```python
from build123d import *

# Parameters (mm, degrees)
SKETCH1_W           = 12
SKETCH1_H           = 12
BOSS_EXTRUDE1_DEPTH = 3
SHELL2_T            = -1.8
SKETCH3_R           = 1.5
CUT_EXTRUDE3_DEPTH  = 1.8
BOSS_EXTRUDE2_START = 2
SKETCH3_3_W         = 16
SKETCH3_3_H         = 16
SKETCH3_3_W_2       = 12
SKETCH3_3_H_2       = 12
SKETCH3_3_R         = 1.5
BOSS_EXTRUDE2_DEPTH = 2
SKETCH4_W           = 14
SKETCH4_H           = 2
BOSS_EXTRUDE3_DEPTH = 2
SKETCH5_W           = 16
SKETCH5_H           = 16
SKETCH5_W_2         = 12
SKETCH5_H_2         = 12
BOSS_EXTRUDE4_DEPTH = 3
SKETCH6_W           = 14
SKETCH6_H           = 5
CUT_EXTRUDE4_DEPTH  = 2
SKETCH7_W           = 12
SKETCH7_H           = 5
CUT_EXTRUDE5_DEPTH  = 2
CUT_EXTRUDE6_DEPTH  = 0.5
SKETCH9_R           = 0.8
CUT_EXTRUDE7_DEPTH  = 21.420577881


with BuildPart() as part:
    # Sketch1 → Boss-Extrude1 (new body)
    with BuildSketch(Plane(origin=(0, 0, 0), x_dir=(1, 0, 0), z_dir=(0, 1, 0))):
        with Locations((6, -6)):
            Rectangle(SKETCH1_W, SKETCH1_H)
    extrude(amount=-BOSS_EXTRUDE1_DEPTH)

    # Shell2
    shell2_openings = [part.faces().sort_by_distance(p)[0] for p in [
        (6, -3, 6),
    ]]
    offset(amount=SHELL2_T, openings=shell2_openings, kind=Kind.INTERSECTION)

    # Sketch3 → Cut-Extrude3 (cut)
    with BuildSketch(Plane(origin=(0, 0, 0), x_dir=(1, 0, 0), z_dir=(0, 1, 0))):
        with Locations(Location((6, -6, 0), (0, 0, 270))):
            Circle(SKETCH3_R)
    extrude(amount=-CUT_EXTRUDE3_DEPTH, mode=Mode.SUBTRACT)

    # Sketch3<3> → Boss-Extrude2 (add)
    # profile 1 of 2: a face of its own
    with BuildSketch(Plane(origin=(0, 0, 0), x_dir=(1, 0, 0), z_dir=(0, 1, 0)).offset(BOSS_EXTRUDE2_START)):
        with Locations((6, -6)):
            Rectangle(SKETCH3_3_W, SKETCH3_3_H)
        with Locations((6, -6)):
            Rectangle(SKETCH3_3_W_2, SKETCH3_3_H_2, mode=Mode.SUBTRACT)
    # profile 2 of 2: a face of its own
    with BuildSketch(Plane(origin=(0, 0, 0), x_dir=(1, 0, 0), z_dir=(0, 1, 0)).offset(BOSS_EXTRUDE2_START)):
        with Locations((6, -6)):
            Rectangle(SKETCH3_3_W_2, SKETCH3_3_H_2)
        with Locations(Location((6, -6, 0), (0, 0, 270))):
            Circle(SKETCH3_3_R, mode=Mode.SUBTRACT)
    extrude(amount=-BOSS_EXTRUDE2_DEPTH)

    # Sketch4 → Boss-Extrude3 (add)
    with BuildSketch(Plane(origin=(0, 2, 0), x_dir=(1, 0, 0), z_dir=(0, 1, 0))):
        Polygon((0, 2), (-2, 2), (-2, -14), (0, -14), (0, 0), align=None)
        with Locations((7, 1)):
            Rectangle(SKETCH4_W, SKETCH4_H)
    extrude(amount=BOSS_EXTRUDE3_DEPTH)

    # Sketch5 → Boss-Extrude4 (add)
    with BuildSketch(Plane.XZ):
        with Locations((6, 6)):
            Rectangle(SKETCH5_W, SKETCH5_H)
        with Locations((6, 6)):
            Rectangle(SKETCH5_W_2, SKETCH5_H_2, mode=Mode.SUBTRACT)
    extrude(amount=BOSS_EXTRUDE4_DEPTH)

    # Sketch6 → Cut-Extrude4 (cut)
    with BuildSketch(Plane.XY.offset(14)):
        with Locations((7, -0.5)):
            Rectangle(SKETCH6_W, SKETCH6_H)
    extrude(amount=-CUT_EXTRUDE4_DEPTH, mode=Mode.SUBTRACT)

    # Sketch7 → Cut-Extrude5 (cut)
    with BuildSketch(Plane(origin=(14, 0, 0), x_dir=(0, 0, -1), z_dir=(1, 0, 0))):
        with Locations((-6, -0.5)):
            Rectangle(SKETCH7_W, SKETCH7_H)
    extrude(amount=-CUT_EXTRUDE5_DEPTH, mode=Mode.SUBTRACT)

    # Sketch8 → Cut-Extrude6 (cut)
    with BuildSketch(Plane.XY.offset(12)):
        with BuildLine():
            Line((5.499365182, -0.030316533), (6.944147055, 0.139116978))
            add(Edge.make_bspline(
                [(6.944147055, 0.139116978), (7.033959338, 0.149589911), (7.207292534, 0.169802147), (7.456935343, 0.206659273), (7.686554115, 0.246864239), (7.896440991, 0.291462829), (8.086108286, 0.339865769), (8.256388111, 0.390049541), (8.406137381, 0.446305372), (8.496905896, 0.49005931), (8.539974305, 0.51081995)],
                knots=[0, 0, 0, 0, 1.318163599, 2.543989528, 3.678365744, 4.716171039, 5.671329954, 6.531514493, 7.303223867, 8, 8, 8, 8], degree=3))
            Line((8.539974305, 0.51081995), (8.894602583, 0.146997606))
            add(Edge.make_bspline(
                [(8.894602583, 0.146997606), (8.903504519, 0.13774703), (8.91939642, 0.121232731), (8.933040884, 0.094560662), (8.942770969, 0.072093955), (8.937635666, 0.051580559), (8.925089845, 0.034251106), (8.900964781, 0.024529461), (8.870149866, 0.016869042), (8.846087974, 0.015236889), (8.832870994, 0.014340361)],
                knots=[0, 0, 0, 0, 1.361923056, 2.431330196, 3.216705747, 3.88751825, 4.590291911, 5.428398407, 6.587442422, 8, 8, 8, 8], degree=3))
            Line((8.832870994, 0.014340361), (8.478242716, -0.021122466))
            Line((8.478242716, -0.021122466), (7.485283538, -0.136705016))
            Line((7.485283538, -0.136705016), (5.934113182, -0.321899783))
            add(Edge.make_bspline(
                [(5.934113182, -0.321899783), (5.850481605, -0.332333939), (5.69237844, -0.352059419), (5.468673749, -0.381100719), (5.271621052, -0.407112207), (5.100999285, -0.431234493), (4.956401672, -0.450505772), (4.838594823, -0.467397889), (4.747497081, -0.481707682), (4.65962381, -0.49747077), (4.562769862, -0.520689248), (4.443406404, -0.552923227), (4.314473425, -0.598718655), (4.224826658, -0.63258625), (4.178046488, -0.6502593)],
                knots=[0, 0, 0, 0, 1.692798098, 3.200187617, 4.530910958, 5.684993954, 6.661249462, 7.46089318, 8.075318241, 8.513415889, 9.253600346, 10.074996663, 10.995479859, 12, 12, 12, 12], degree=3))
            Line((4.178046488, -0.6502593), (3.85100041, -0.366556678))
            add(Edge.make_bspline(
                [(3.85100041, -0.366556678), (3.838610297, -0.356171923), (3.812805776, -0.334543902), (3.803900048, -0.290524917), (3.80934915, -0.25628733), (3.825603847, -0.233888183), (3.853323458, -0.221153848), (3.874526491, -0.217543712), (3.886463237, -0.2155113)],
                knots=[0, 0, 0, 0, 1.325695646, 2.760987115, 3.510625552, 4.19429037, 4.983433253, 6, 6, 6, 6], degree=3))
            Line((3.886463237, -0.2155113), (4.276554343, -0.180048472))
            Line((4.276554343, -0.180048472), (5.499365182, -0.030316533))
        make_face()
    extrude(amount=-CUT_EXTRUDE6_DEPTH, mode=Mode.SUBTRACT)

    # Sketch9 → Cut-Extrude7 (cut, through all)
    with BuildSketch(Plane(origin=(0, 2, 0), x_dir=(1, 0, 0), z_dir=(0, 1, 0))):
        with Locations(Location((2, -10, 0), (0, 0, 270))):
            Circle(SKETCH9_R)
        with Locations(Location((10, -10, 0), (0, 0, 270))):
            Circle(SKETCH9_R)
        with Locations(Location((2, -2, 0), (0, 0, 270))):
            Circle(SKETCH9_R)
        with Locations(Location((10, -2, 0), (0, 0, 270))):
            Circle(SKETCH9_R)
    extrude(amount=-CUT_EXTRUDE7_DEPTH, mode=Mode.SUBTRACT)


solid = part.part
```
Can you work these out from the model? Positions are in its coordinate system, mm. A direction names the side the tool comes from. Coordinates: 2 decimals unless noted, no trailing zeros. Loops run counter-clockwise (first coordinate to the right, second up) from the corner with the lowest first, then second, coordinate; pieces in that order, holes last. Notation, with made-up numbers: (-22.5, -34.75) -> (8.5, -34.75) arc R30 ccw to (8.5, -4.75) -> close; hole circle Ø6 at (-7, 69). An arc over 180 degrees is marked (long way). Answer as a JSON object with one key per item and string values.
1) Imagine slicing it at A-A (x = 10). Please give me the cut outline in (y, z), then the cut area to 3 significant figures.
Results:
{"outline": "(-3, -2) -> (4, -2) -> (4, 0) -> (2, 0) -> (2, 1.2) -> (-3, 1.2) -> close; (-3, 10.8) -> (2, 10.8) -> (2, 12) -> (-3, 12) -> close; (-1.8, 2.8) -> (2, 2.8) -> (2, 9.2) -> (-1.8, 9.2) -> close", "area": "50.3 mm^2"}
2) Imagine slicing it at C-C (z = 10). Please give me the cut outline in (x, y).
Results:
{"outline": "(-2, -3) -> (1.2, -3) -> (1.2, 2) -> (0, 2) -> (0, 4) -> (-2, 4) -> close; (2.8, -1.8) -> (9.2, -1.8) -> (9.2, 2) -> (2.8, 2) -> close; (10.8, -3) -> (12, -3) -> (12, 2) -> (10.8, 2) -> close"}
3) If I drill on line 1 (X direction, y = 0.5, z = 2); line 2 (X direction, y = 0, z = 6), over which ranges is the centre line in solid material (lowest first)?
Results:
{"line 1": "x = -2 to 1.2, 2.8 to 9.2, 10.8 to 12", "line 2": "x = -2 to 4.5, 7.5 to 12"}
4) Imagine slicing it at B-B (z = 6). Please give me the cut outline in (x, y), then the cut area to 3 significant figures.
Results:
{"outline": "(-2, -3) -> (1.8, -3) -> (1.8, -1.8) -> (4.5, -1.8) -> (4.5, 2) -> (0, 2) -> (0, 4) -> (-2, 4) -> close; (7.5, -1.8) -> (10.2, -1.8) -> (10.2, -3) -> (12, -3) -> (12, 2) -> (7.5, 2) -> close", "area": "52.5 mm^2"}
5) For P1, Ø3.5, axis at y = 0, z = 9, coming from the +X side; P2, Ø1.3, axis at x = 6, y = 0, coming from the +Z side; P3, Ø1.4, axis at x = 10, z = 10, coming from the +Y side; P4, Ø6.5, axis at x = 5.5, z = 5.5, coming from the -Y side, each with a flat end and sliding along its axis, tell me the tip position at first contact or that it passes through.
Results:
{"P1": "stops at x = 12", "P2": "stops at z = 12", "P3": "passes through", "P4": "stops at y = -1.8"}
6) Thinking about a two-plate mould opening in Z: for faces 5 (the face through (6.4, -0.1, 11.5)), 6 (the face through (6, -2, 10.2)), 7 (the face through (0, 3, 9)), 8 (the face through (6, 1, -2)), which applies, pulls with the +Z half, pulls with the -Z half, needs draft (parallel to the pull), parting line crosses it, or undercut?
Results:
{"face 5": "pulls with the +Z half", "face 6": "undercut", "face 7": "needs draft", "face 8": "pulls with the -Z half"}
7) For faces 1 (the face through (12, 0, 6)), 2 (the face through (4.6, 2, 4.6)), 3 (the face through (1.51, -0.46, 1.37)), 4 (the face through (6, -1.8, 4)), which set-ups out of +Z, -Z, +X, -X, +Y, -Y let a thin tool reach every point of the face, with its end or its side?
Results:
{"face 1": "+Z, +X, +Y, -Y", "face 2": "+Z, +X, +Y", "face 3": "+Y, -Y", "face 4": "-Y"}
8) Imagine slicing it at D-D (y = 3). Please give me the cut outline in (x, z), then the cut area to 3 significant figures.
Results:
{"outline": "(-2, -2) -> (14, -2) -> (14, 0) -> (0, 0) -> (0, 14) -> (-2, 14) -> close", "area": "60.0 mm^2"}
